```python
from build123d import *

# Parameters (mm, degrees)
SKETCH031_W          = 70.7
SKETCH031_H          = 95.7
PAD016_DEPTH         = 47.6
THICKNESS016_T       = -1.6
POCKET015_DEPTH      = 47.851
POCKET015_DEPTH_BACK = 47.851
POCKET016_DEPTH      = 35.351
POCKET016_DEPTH_BACK = 35.351
SKETCH034_R          = 10.125
POCKET017_DEPTH      = 0.001
POCKET017_DEPTH_BACK = 47.601
FILLET002_R          = 4


with BuildPart() as part:
    # Sketch031 → Pad016 (new body)
    with BuildSketch(Plane.XY):
        Rectangle(SKETCH031_W, SKETCH031_H)
    extrude(amount=PAD016_DEPTH)

    # Thickness016
    thickness016_openings = [part.faces().sort_by_distance(p)[0] for p in [
        (0, 0, 47.6),
    ]]
    offset(amount=THICKNESS016_T, openings=thickness016_openings, kind=Kind.INTERSECTION)

    # Sketch032 → Pocket015 (cut, two sides)
    with BuildSketch(Plane.XZ) as pocket015_sk:
        with BuildLine():
            Line((-23.35, 47.6), (23.35, 47.6))
            Line((23.35, 47.6), (23.35, 20))
            ThreePointArc((15.35, 12), (21.006854, 14.343146), (23.35, 20))
            Line((15.35, 12), (-15.35, 12))
            ThreePointArc((-23.35, 20), (-21.006854, 14.343146), (-15.35, 12))
            Line((-23.35, 20), (-23.35, 47.6))
        make_face()
    extrude(amount=-POCKET015_DEPTH, mode=Mode.SUBTRACT)
    extrude(pocket015_sk.sketch, amount=POCKET015_DEPTH_BACK, mode=Mode.SUBTRACT)

    # Sketch033 → Pocket016 (cut, two sides)
    with BuildSketch(Plane.YZ) as pocket016_sk:
        with BuildLine():
            Line((-35.85, 47.6), (35.85, 47.6))
            Line((35.85, 47.6), (35.85, 20))
            ThreePointArc((27.85, 12), (33.506854, 14.343146), (35.85, 20))
            Line((27.85, 12), (-27.85, 12))
            ThreePointArc((-35.85, 20), (-33.506854, 14.343146), (-27.85, 12))
            Line((-35.85, 20), (-35.85, 47.6))
        make_face()
    extrude(amount=-POCKET016_DEPTH, mode=Mode.SUBTRACT)
    extrude(pocket016_sk.sketch, amount=POCKET016_DEPTH_BACK, mode=Mode.SUBTRACT)

    # Sketch034 → Pocket017 (cut, two sides)
    with BuildSketch(Plane.XY) as pocket017_sk:
        with Locations((0, 47.85)):
            Circle(SKETCH034_R)
        with Locations((0, -47.85)):
            Circle(SKETCH034_R)
        with Locations((35.35, 0)):
            Circle(SKETCH034_R)
        with Locations((-35.35, 0)):
            Circle(SKETCH034_R)
        with BuildLine():
            ThreePointArc((10.125, 10.125), (0, 20.25), (-10.125, 10.125))
            Line((-10.125, 10.125), (-10.125, -10.125))
            ThreePointArc((-10.125, -10.125), (0, -20.25), (10.125, -10.125))
            Line((10.125, 10.125), (10.125, -10.125))
        make_face()
    extrude(amount=-POCKET017_DEPTH, mode=Mode.SUBTRACT)
    extrude(pocket017_sk.sketch, amount=POCKET017_DEPTH_BACK, mode=Mode.SUBTRACT)

    # Fillet002
    fillet002_edges = [part.edges().sort_by_distance(p)[0] for p in [
        (34.547475, -10.093145, 12),
        (34.547475, 10.093145, 12),
        (34.55, 35.85, 47.6),
        (23.35, 47.05, 47.6),
        (10.093145, 47.047475, 12),
        (-10.093145, 47.047475, 12),
        (-23.35, 47.05, 47.6),
        (-34.55, 35.85, 47.6),
        (-34.547475, 10.093145, 12),
        (-34.547475, -10.093145, 12),
        (-34.55, -35.85, 47.6),
        (-23.35, -47.05, 47.6),
        (-10.093145, -47.047475, 12),
        (10.093145, -47.047475, 12),
        (23.35, -47.05, 47.6),
        (34.55, -35.85, 47.6),
    ]]
    fillet(fillet002_edges, radius=FILLET002_R)


with BuildPart() as part_1:
    # Body016 placement: moved
    add(part.part.moved(Location((69.1, 0, 0))))


solid = part_1.part
```
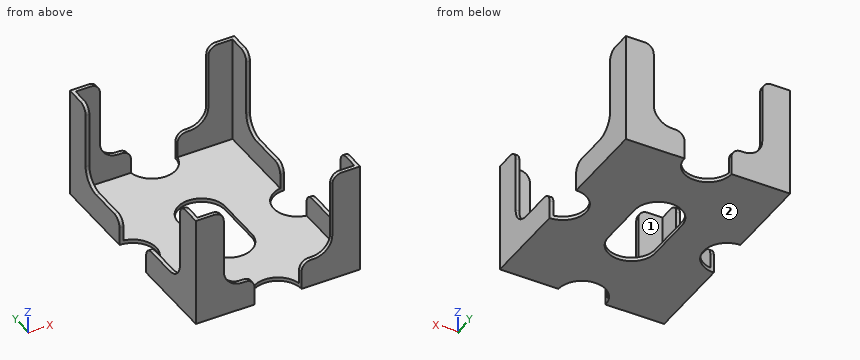
The listing builds one solid part. Answer for the finished solid, in the listing's coordinates (mm). Face numbers are marked on the shaded views. A direction names the side the tool comes from. Coordinates: 2 decimals unless noted, no trailing zeros. Loops run counter-clockwise (first coordinate to the right, second up) from the corner with the lowest first, then second, coordinate; pieces in that order, holes last. Notation, with made-up numbers: (14, 45.5) -> (39, 45.5) arc R7 cw to (39, 53.5) -> close; hole circle Ø6 at (5.25, -33). An arc over 180 degrees is marked (long way). Return JSON: item names as keys, results as strings. Group by question number.
(1) Find the intervals of material crossed by probe 1 along Y at (x, z) = (92, 11); probe 2 along X at (y, z) = (-40.5, 6), in increasing order. Write a range as from..to.
(2) A cutting plane is placed at B-B on y = 0. Write down the section's boundary in (x, z) (3 decimals).
(3) Given pin 1 Ø0.5 at (y, z) = (-4, 0.5) entering from +X; pin 2 Ø1.1 at (x, y) = (84, -47) entering from +Z; pin 3 Ø7 at (x, z) = (85.5, 18.5) entering from +Y; pin 4 Ø10 at (x, y) = (53.5, -29.5) entering from +Z, each flat-ended and moving along its own axis, determine where each tip first touches the part or whether it passes through.
(4) Which of the six approach directions +Z, -Z, +X, -X, +Y, -Y give full straight-line access (tool end or side, diameter ignored) to the marked faces 1 and 2?
(5) A cutting plane is placed at C-C on x = 69.1. Write down the section's boundary in (y, z) (3 decimals).
(6) A cutting plane is placed at A-A on z = 22. Write down the section's boundary in (x, y), and give its area (3 significant figures).
(7) A cutting plane is placed at D-D on y = -41. Write down the section's boundary in (x, z), and give its area (3 significant figures).
The answers:
{
 "1": {"probe 1": "y = -47.85..-46.25, 46.25..47.85", "probe 2": "x = 33.75..35.35, 102.85..104.45"},
 "2": {"outline": "(43.875, 0) -> (58.975, 0) -> (58.975, 1.6) -> (43.875, 1.6) -> close; (79.225, 0) -> (94.325, 0) -> (94.325, 1.6) -> (79.225, 1.6) -> close"},
 "3": {"pin 1": "stops at x = 95.26", "pin 2": "stops at z = 12", "pin 3": "passes through", "pin 4": "stops at z = 1.6"},
 "4": {"face 1": "+Z", "face 2": "-Z, +X, -X, +Y, -Y"},
 "5": {"outline": "(-37.725, 0) -> (-20.25, 0) -> (-20.25, 1.6) -> (-37.725, 1.6) -> close; (20.25, 0) -> (37.725, 0) -> (37.725, 1.6) -> (20.25, 1.6) -> close"},
 "6": {"outline": "(33.75, -47.85) -> (45.75, -47.85) -> (45.75, -46.25) -> (35.35, -46.25) -> (35.35, -35.85) -> (33.75, -35.85) -> close; (33.75, 35.85) -> (35.35, 35.85) -> (35.35, 46.25) -> (45.75, 46.25) -> (45.75, 47.85) -> (33.75, 47.85) -> close; (92.45, -47.85) -> (104.45, -47.85) -> (104.45, -35.85) -> (102.85, -35.85) -> (102.85, -46.25) -> (92.45, -46.25) -> close; (92.45, 46.25) -> (102.85, 46.25) -> (102.85, 35.85) -> (104.45, 35.85) -> (104.45, 47.85) -> (92.45, 47.85) -> close", "area": "143 mm^2"},
 "7": {"outline": "(33.75, 0) -> (61.64, 0) -> (61.64, 1.6) -> (35.35, 1.6) -> (35.35, 47.6) -> (33.75, 47.6) -> close; (76.56, 0) -> (104.45, 0) -> (104.45, 47.6) -> (102.85, 47.6) -> (102.85, 1.6) -> (76.56, 1.6) -> close", "area": "236 mm^2"}
}
